```python
from build123d import *

# Parameters (mm, degrees)
BOSS_EXTRUDE2_DEPTH     = 6.35
CUT_EXTRUDE1_DEPTH      = 198.667656687
CUT_EXTRUDE1_DEPTH_BACK = 198.667656687
SKETCH2_R               = 5.55625
CUT_EXTRUDE2_DEPTH      = 198.667656687
CUT_EXTRUDE2_DEPTH_BACK = 1.5875
SKETCH3_W               = 1.5875
SKETCH3_H               = 87.3
SKETCH3_3_R             = 3.175
BOSS_EXTRUDE3_DEPTH     = 4.7625
SKETCH6_R               = 14
BOSS_EXTRUDE7_DEPTH     = 8
BOSS_EXTRUDE8_START     = -139.7
BOSS_EXTRUDE8_DEPTH     = 12.7
BOSS_EXTRUDE9_START     = 50.8
SKETCH12_R              = 4.7625
BOSS_EXTRUDE9_DEPTH     = 50.8
SKETCH13_R              = 14
CUT_EXTRUDE3_DEPTH      = 8


with BuildPart() as part:
    # Sketch1 → Boss-Extrude2 (new body)
    with BuildSketch(Plane.XY):
        with BuildLine():
            Line((-25.4, 0), (-114.3, 0))
            ThreePointArc((-114.3, 0), (-132.260512242, -7.439487758), (-139.7, -25.4))
            Line((-139.7, -25.4), (-139.7, -114.3))
            ThreePointArc((-139.7, -114.3), (-132.260512242, -132.260512242), (-114.3, -139.7))
            Line((-114.3, -139.7), (-25.4, -139.7))
            ThreePointArc((-25.4, -139.7), (-7.439487758, -132.260512242), (0, -114.3))
            Line((0, -114.3), (0, -25.4))
            ThreePointArc((0, -25.4), (-7.439487758, -7.439487758), (-25.4, 0))
        make_face()
    extrude(amount=BOSS_EXTRUDE2_DEPTH)

    # Sketch2 → Cut-Extrude1 (cut, two sides: drawn at the far end of the back side and taken through both)
    with BuildSketch(Plane.XY.offset(6.35).offset(-CUT_EXTRUDE1_DEPTH_BACK)):
        with Locations((-69.85, -69.85)):
            Circle(SKETCH2_R)
        with BuildLine():
            Line((-95.602147834, -25.4), (-44.097852166, -25.4))
            ThreePointArc((-44.097852166, -25.4), (-38.231217135, -29.319960204), (-39.607724106, -36.240128061))
            Line((-39.607724106, -36.240128061), (-60.869743879, -57.502147834))
            ThreePointArc((-60.869743879, -57.502147834), (-69.85, -61.221891712), (-78.830256121, -57.502147834))
            Line((-78.830256121, -57.502147834), (-100.092275894, -36.240128061))
            ThreePointArc((-100.092275894, -36.240128061), (-101.468782865, -29.319960204), (-95.602147834, -25.4))
        make_face()
        with BuildLine():
            Line((-57.502147834, -78.830256121), (-36.240128061, -100.092275894))
            ThreePointArc((-36.240128061, -100.092275894), (-29.319960204, -101.468782865), (-25.4, -95.602147834))
            Line((-25.4, -95.602147834), (-25.4, -44.097852166))
            ThreePointArc((-25.4, -44.097852166), (-29.319960204, -38.231217135), (-36.240128061, -39.607724106))
            Line((-36.240128061, -39.607724106), (-57.502147834, -60.869743879))
            ThreePointArc((-57.502147834, -60.869743879), (-61.221891712, -69.85), (-57.502147834, -78.830256121))
        make_face()
        with BuildLine():
            Line((-78.830256121, -82.197852166), (-100.092275894, -103.459871939))
            ThreePointArc((-100.092275894, -103.459871939), (-101.468782865, -110.380039796), (-95.602147834, -114.3))
            Line((-95.602147834, -114.3), (-44.097852166, -114.3))
            ThreePointArc((-44.097852166, -114.3), (-38.231217135, -110.380039796), (-39.607724106, -103.459871939))
            Line((-39.607724106, -103.459871939), (-60.869743879, -82.197852166))
            ThreePointArc((-60.869743879, -82.197852166), (-69.85, -78.478108288), (-78.830256121, -82.197852166))
        make_face()
        with BuildLine():
            Line((-82.197852166, -60.869743879), (-103.459871939, -39.607724106))
            ThreePointArc((-103.459871939, -39.607724106), (-110.380039796, -38.231217135), (-114.3, -44.097852166))
            Line((-114.3, -44.097852166), (-114.3, -95.602147834))
            ThreePointArc((-114.3, -95.602147834), (-110.380039796, -101.468782865), (-103.459871939, -100.092275894))
            Line((-103.459871939, -100.092275894), (-82.197852166, -78.830256121))
            ThreePointArc((-82.197852166, -78.830256121), (-78.478108288, -69.85), (-82.197852166, -60.869743879))
        make_face()
    extrude(amount=CUT_EXTRUDE1_DEPTH + CUT_EXTRUDE1_DEPTH_BACK, mode=Mode.SUBTRACT)

    # Sketch3 → Cut-Extrude2 (cut, two sides: drawn at the far end of the back side and taken through both)
    with BuildSketch(Plane.XY.offset(6.35).offset(-CUT_EXTRUDE2_DEPTH_BACK)):
        Polygon((-26.2, -119.05625), (-69.85, -119.05625), (-113.5, -119.05625), (-113.5, -120.64375), (-26.2, -120.64375), align=None)
        Polygon((-29.391522129, -28.268990114), (-69.85, -68.727467985), (-68.727467985, -69.85), (-28.268990114, -29.391522129), align=None)
        Polygon((-70.972532015, -69.85), (-69.85, -68.727467985), (-110.308477871, -28.268990114), (-111.431009886, -29.391522129), align=None)
        Polygon((-113.5, -20.64375), (-69.85, -20.64375), (-26.2, -20.64375), (-26.2, -19.05625), (-113.5, -19.05625), align=None)
        Polygon((-110.308477871, -111.431009886), (-69.85, -70.972532015), (-70.972532015, -69.85), (-111.431009886, -110.308477871), align=None)
        Polygon((-68.727467985, -69.85), (-69.85, -70.972532015), (-29.391522129, -111.431009886), (-28.268990114, -110.308477871), align=None)
        with Locations((-119.85, -69.85)):
            Rectangle(SKETCH3_W, SKETCH3_H)
        with Locations((-19.85, -69.85)):
            Rectangle(SKETCH3_W, SKETCH3_H)
    extrude(amount=CUT_EXTRUDE2_DEPTH + CUT_EXTRUDE2_DEPTH_BACK, mode=Mode.SUBTRACT)

    # Sketch3<3> → Boss-Extrude3 (add)
    with BuildSketch(Plane.XY.offset(6.35)):
        with Locations(Location((-119.85, -19.85, 0), (0, 0, 180))):
            Circle(SKETCH3_3_R)
        with Locations(Location((-19.85, -19.85, 0), (0, 0, 180))):
            Circle(SKETCH3_3_R)
        with Locations(Location((-19.85, -119.85, 0), (0, 0, 180))):
            Circle(SKETCH3_3_R)
        with Locations(Location((-119.85, -119.85, 0), (0, 0, 180))):
            Circle(SKETCH3_3_R)
    extrude(amount=BOSS_EXTRUDE3_DEPTH)

    # Sketch6 → Boss-Extrude7 (add)
    with BuildSketch(Plane(origin=(0, 0, 0), x_dir=(1, 0, 0), z_dir=(0, 1, 0))):
        with BuildLine():
            Line((-98.1375, -6.35), (-90.771408037, -6.35))
            ThreePointArc((-90.771408037, -6.35), (-89.338621713, -3.021552737), (-87.338207531, 0))
            Line((-87.338207531, 0), (-90.145452854, 0))
            ThreePointArc((-90.145452854, 0), (-87.742009924, 0.472418688), (-85.696183168, 1.819382022))
            ThreePointArc((-85.696183168, 1.819382022), (-71.4375, 7.65), (-57.178816832, 1.819382022))
            ThreePointArc((-57.178816832, 1.819382022), (-55.132990076, 0.472418688), (-52.729547146, 0))
            Line((-52.729547146, 0), (-55.536792469, 0))
            ThreePointArc((-55.536792469, 0), (-53.536378287, -3.021552737), (-52.103591963, -6.35))
            Line((-52.103591963, -6.35), (-44.7375, -6.35))
            ThreePointArc((-44.7375, -6.35), (-49.227628061, -8.209871939), (-51.0875, -12.7))
            ThreePointArc((-51.0875, -12.7), (-71.4375, -33.05), (-91.7875, -12.7))
            ThreePointArc((-91.7875, -12.7), (-93.647371939, -8.209871939), (-98.1375, -6.35))
        make_face()
        with Locations((-71.4375, -12.7)):
            Circle(SKETCH6_R, mode=Mode.SUBTRACT)
    extrude(amount=-BOSS_EXTRUDE7_DEPTH)

    # Sketch5 → Boss-Extrude8 (add)
    with BuildSketch(Plane(origin=(0, 0, 0), x_dir=(1, 0, 0), z_dir=(0, 1, 0)).offset(BOSS_EXTRUDE8_START)):
        with BuildLine():
            Line((-82.55, -6.35), (-60.325, -6.35))
            ThreePointArc((-60.325, -6.35), (-64.815128061, -8.209871939), (-66.675, -12.7))
            ThreePointArc((-66.675, -12.7), (-71.4375, -17.4625), (-76.2, -12.7))
            ThreePointArc((-76.2, -12.7), (-78.059871939, -8.209871939), (-82.55, -6.35))
        make_face()
    extrude(amount=BOSS_EXTRUDE8_DEPTH)

    # Sketch12 → Boss-Extrude9 (add)
    with BuildSketch(Plane.XZ.offset(139.7).offset(BOSS_EXTRUDE9_START)):
        with Locations((-71.4375, 12.7)):
            Circle(SKETCH12_R)
    extrude(amount=-BOSS_EXTRUDE9_DEPTH)

    # Sketch13 → Cut-Extrude3 (cut)
    with BuildSketch(Plane(origin=(0, 0, 0), x_dir=(1, 0, 0), z_dir=(0, 1, 0))):
        with Locations(Location((-71.4375, -12.7, 0), (0, 0, 270))):
            Circle(SKETCH13_R)
    extrude(amount=-CUT_EXTRUDE3_DEPTH, mode=Mode.SUBTRACT)


solid = part.part
```
Input: part model. Units: mm. Frame: model coordinates. A direction names the side the tool comes from. Give positions to 0.01 mm unless a question says otherwise; leave off trailing zeros. Order: outer loops, then holes, each group sorted by start corner. A loop starts at its lowest first (then second) coordinate and runs counter-clockwise, first axis right, second up. Notation, with made-up numbers: (80, 76.25) - (139, 76.25) arc R16 cw to (139, 81.25) - close; hole circle Ø4 at (51.5, 43). An arc over 180 degrees is marked (long way). Use a Markdown table: item, result.
(1) Draft query along Y for faces 1 (the flat face through (0, -70, 3)), 2 (the cylindrical face through (-132.06, -7.24, 3.13)), 3 (the cylindrical face through (-29.224, -38.272, 3.131)). Return one class per face: released by +Y, released by -Y, zero draft, split by the parting line, or undercut.
Computed values:
| item | result |
|---|---|
| face 1 | zero draft |
| face 2 | released by +Y |
| face 3 | undercut |
(2) Access query for faces 4 (the flat face through (-71, -127, 11)), 5 (the cylindrical face through (-61.22, -69.71, 3.13)), 6 (the flat face through (-93.125, -47.697, 5.545)). Directions: +Z, -Z, +X, -X, +Y, -Y. A direction counts if a zero-diameter tool reaches every point of the face in a straight line with its end or side. Return the directions, or none.
Computed values:
| item | result |
|---|---|
| face 4 | +Z, +X, -X, +Y |
| face 5 | +Z, -Z |
| face 6 | +Z |
(3) Section query C-C (x = -32.5). Output: boundary loops of the cut face in (y, z), then the cut area to 3 significant figures.
Computed values:
| item | result |
|---|---|
| outline | (-139.7, 0) - (-101.91, 0) - (-101.91, 6.35) - (-106.08, 6.35) - (-106.08, 4.76) - (-108.32, 4.76) - (-108.32, 6.35) - (-119.06, 6.35) - (-119.06, 4.76) - (-120.64, 4.76) - (-120.64, 6.35) - (-139.7, 6.35) - close; (-37.79, 0) - (0, 0) - (0, 6.35) - (-19.06, 6.35) - (-19.06, 4.76) - (-20.64, 4.76) - (-20.64, 6.35) - (-31.38, 6.35) - (-31.38, 4.76) - (-33.62, 4.76) - (-33.62, 6.35) - (-37.79, 6.35) - close |
| area | 468 mm2 |
(4) Section query A-A (z = 24). Output: boundary loops of the cut face in (x, y).
Computed values:
| item | result |
|---|---|
| outline | (-88.36, -8) - (-79.7, -8) - (-79.7, 0) - (-88.36, 0) - close; (-63.17, -8) - (-54.51, -8) - (-54.51, 0) - (-63.17, 0) - close |
(5) Section query D-D (x = -69.85). State how many separate pieces and enclosed holes the cut face has, then the cut area to 3 significant figures.
Computed values:
| item | result |
|---|---|
| separate pieces | 6 |
| enclosed holes | 0 |
| area | 1,000 mm2 |
(6) Section query B-B (y = -69.85). Output: boundary loops of the cut face in (x, z), then the cut area to 3 significant figures.
Computed values:
| item | result |
|---|---|
| outline | (-139.7, 0) - (-114.3, 0) - (-114.3, 6.35) - (-119.06, 6.35) - (-119.06, 4.76) - (-120.64, 4.76) - (-120.64, 6.35) - (-139.7, 6.35) - close; (-78.48, 0) - (-75.41, 0) - (-75.41, 6.35) - (-78.48, 6.35) - close; (-64.29, 0) - (-61.22, 0) - (-61.22, 6.35) - (-64.29, 6.35) - close; (-25.4, 0) - (0, 0) - (0, 6.35) - (-19.06, 6.35) - (-19.06, 4.76) - (-20.64, 4.76) - (-20.64, 6.35) - (-25.4, 6.35) - close |
| area | 357 mm2 |
(7) Line query: line 1 (X direction, y = -69.85, z = 1.75); line 2 (X direction, y = -50, z = 4.5); line 3 (Y direction, x = -98, z = 2.5). Output: solid intervals per line, ascending. Write a range as from..to.
Computed values:
| item | result |
|---|---|
| line 1 | x = -139.7..-114.3, -78.48..-75.41, -64.29..-61.22, -25.4..0 |
| line 2 | x = -139.7..-114.3, -93.07..-86.33, -53.37..-46.63, -25.4..0 |
| line 3 | y = -139.7..-113.83, -101.37..-94.63, -45.07..-38.33, -25.87..0 |
(8) Pin query (flat end, axial travel): pin 1 (12 mm diameter, centred on x = -17, z = -1, fed in from -Y); pin 2 (12 mm diameter, centred on x = -32, z = 12.5, fed in from +Y); pin 3 (0.8 mm diameter, centred on x = -63.5, z = 5, fed in from -Y); pin 4 (1.3 mm diameter, centred on x = -20, z = 5.5, fed in from +Y). Return the tip coordinate at first contact, or that it passes through.
Computed values:
| item | result |
|---|---|
| pin 1 | stops at y = -139.58 |
| pin 2 | passes through |
| pin 3 | stops at y = -139.7 |
| pin 4 | stops at y = -0.45 |
